```python
from build123d import *

# Parameters (mm, degrees)
F1_DEPTH  = 18
F2_W      = 1
F2_H      = 18
F3_DEPTH  = 2
F4_W      = 1
F4_H      = 18
F5_DEPTH  = 2
F6_W      = 1
F6_H      = 18
F7_DEPTH  = 2
F8_W      = 1
F8_H      = 18
F9_DEPTH  = 2
F10_W     = 1
F10_H     = 18
F11_DEPTH = 2


with BuildPart() as f1:
    # F0 (on Top) → F1 (new body)
    with BuildSketch(Plane.XY):
        Polygon((0, -10.3779398619), (9.8700073314, -3.2069597839), (6.1, 8.3959297149), (-6.1, 8.3959297149), (-9.8700073314, -3.2069597839), align=None)
        Polygon((-5.9933346782, -1.947352483), (-3.7040845371, 5.0982349887), (3.7040845371, 5.0982349887), (5.9933346782, -1.947352483), (0, -6.3017650113), align=None, mode=Mode.SUBTRACT)
    extrude(amount=F1_DEPTH)

    # F2 (on face) → F3 (join)
    with BuildSketch(Plane(origin=(4.9350036657, -6.7924498229, 0), x_dir=(0.8090169944, 0.5877852523, 0), z_dir=(0.5877852523, -0.8090169944, 0))):
        with Locations((-5.6, 9)):
            Rectangle(F2_W, F2_H)
        with Locations((5.6, 9)):
            Rectangle(F2_W, F2_H)
    extrude(amount=F3_DEPTH)

    # F4 (on face) → F5 (join)
    with BuildSketch(Plane(origin=(-4.9350036657, -6.7924498229, 0), x_dir=(0.8090169944, -0.5877852523, 0), z_dir=(-0.5877852523, -0.8090169944, 0))):
        with Locations((5.6, 9)):
            Rectangle(F4_W, F4_H)
        with Locations((-5.6, 9)):
            Rectangle(F4_W, F4_H)
    extrude(amount=F5_DEPTH)

    # F6 (on face) → F7 (join)
    with BuildSketch(Plane(origin=(-7.9850036657, 2.5944849655, 0), x_dir=(-0.3090169944, -0.9510565163, 0), z_dir=(-0.9510565163, 0.3090169944, 0))):
        with Locations((5.6, 9)):
            Rectangle(F6_W, F6_H)
        with Locations((-5.6, 9)):
            Rectangle(F6_W, F6_H)
    extrude(amount=F7_DEPTH)

    # F8 (on face) → F9 (join)
    with BuildSketch(Plane(origin=(7.9850036657, 2.5944849655, 0), x_dir=(-0.3090169944, 0.9510565163, 0), z_dir=(0.9510565163, 0.3090169944, 0))):
        with Locations((-5.6, 9)):
            Rectangle(F8_W, F8_H)
        with Locations((5.6, 9)):
            Rectangle(F8_W, F8_H)
    extrude(amount=F9_DEPTH)

    # F10 (on face) → F11 (join)
    with BuildSketch(Plane(origin=(0, 8.3959297149, 0), x_dir=(-1, 0, 0), z_dir=(0, 1, 0))):
        with Locations((5.6, 9)):
            Rectangle(F10_W, F10_H)
        with Locations((-5.6, 9)):
            Rectangle(F10_W, F10_H)
    extrude(amount=F11_DEPTH)


solid = f1.part
```
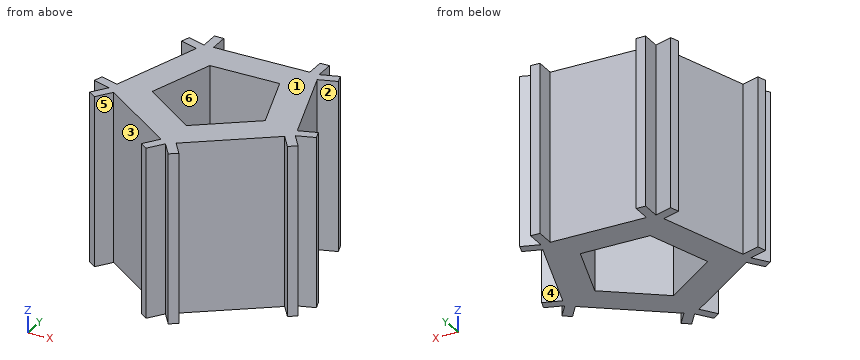
Read the model definition and answer for the solid it produces. Units are mm, in the model's axes. Face numbers are marked on the shaded views. A direction names the side the tool comes from. Round coordinates to 2 decimals unless told otherwise and drop trailing zeros. Write each loop counter-clockwise with the first axis right and the second up, starting at its lowest first coordinate (ties: lowest second). Pieces come first, ordered by that corner, then holes. Notation, with made-up numbers: M 89.5,62 L 114.5,62 A8 ccw 114.5,74 Z; hole C 84,41.5 d10. An arc over 180 degrees is marked long. One line per item, written item: value.
Q1. Straight lines are drawn through the part: line 1 (Y direction, x = 1, z = 11.75); line 2 (Y direction, x = 1.5, z = 10.5); line 3 (X direction, y = 0, z = 1.5). For each, find the intervals that lie inside material, in ascending order. Write a range as [from, to].
Data:
line 1: [-11.75, -10.05], [-9.65, -5.58], [5.1, 8.4]
line 2: [-11.76, -10.74], [-9.29, -5.21], [5.1, 8.4]
line 3: [-8.83, -5.36], [5.36, 8.83]
Q2. Find section B-B on y = -1.25. Write down the section's boundary in (x, z).
Data:
outline: M -9.23,0 L -5.77,0 L -5.77,18 L -9.23,18 Z; M 5.77,0 L 9.23,0 L 9.23,18 L 5.77,18 Z
Q3. For a pull along X with two mould halves and no side action, classify the marked faces 1, 2 and 3 as +X half, -X half, draft (parallel to the pull), parting line (faces both ways), or undercut.
Data:
face 1: draft
face 2: +X half
face 3: undercut
Q4. Which of the six approach directions +Z, -Z, +X, -X, +Y, -Y give full straight-line access (tool end or side, diameter ignored) to the marked faces 4, 5 and 6?
Data:
face 4: +Z, -Z, +Y
face 5: +Z, -Z, -Y
face 6: +Z, -Z
Q5. Find section C-C on y = -7.5. Write down the section's boundary in (x, z), plus the area to 3 significant figures.
Data:
outline: M -3.96,0 L 3.96,0 L 3.96,18 L -3.96,18 Z
area: 143 mm2
Q6. Flat-ended cylindrical pins translate along their axes: pin 1 Ø4 at (y, z) = (6.5, 11) entering from -X; pin 2 Ø0.6 at (y, z) = (10, 5.5) entering from +X; pin 3 Ø1.5 at (y, z) = (3.5, 5.5) entering from -X. Find the tip coordinate at first contact, or state that the pin passes through.
Data:
pin 1: x = -8.31
pin 2: x = 6.1
pin 3: x = -7.93
Q7. Find section A-A on x = 3. Write down the section's boundary in (y, z), plus the area to 3 significant figures.
Data:
outline: M -8.2,0 L -4.12,0 L -4.12,18 L -8.2,18 Z; M 5.1,0 L 8.4,0 L 8.4,18 L 5.1,18 Z
area: 133 mm2
